from build123d import *

# Parameters (mm, degrees)
SKETCH1_R           = 9.5
BOSS_EXTRUDE1_DEPTH = 2.25


with BuildPart() as part:
    # Sketch1 → Boss-Extrude1 (new body)
    with BuildSketch(Plane(origin=(0, 0, 0), x_dir=(1, 0, 0), z_dir=(0, 1, 0))):
        Circle(SKETCH1_R)
        with BuildLine():
            ThreePointArc((-2.050056302, -4.013405112), (-0.801449739, -2.21696931), (0.006631996, -4.249997556))
            ThreePointArc((0.006631996, -4.249997556), (-1.028537661, -4.191035191), (-2.050056302, -4.013405112))
        make_face(mode=Mode.SUBTRACT)
        with BuildLine():
            ThreePointArc((7.644442426, 0), (5.613326884, -2.284952828), (2.934499964, -3.758155497))
            ThreePointArc((2.934499964, -3.758155497), (0, 3.643549808), (-2.934499964, -3.758155497))
            ThreePointArc((-2.934499964, -3.758155497), (-5.613326884, -2.284952828), (-7.644442426, 0))
            ThreePointArc((-7.644442426, 0), (0, 4.25), (7.644442426, 0))
        make_face(mode=Mode.SUBTRACT)
    extrude(amount=BOSS_EXTRUDE1_DEPTH)


solid = part.part
Geometry: final body of the model. Coordinates: model frame, mm. A direction names the side the tool comes from. Give positions to 0.01 mm unless a question says otherwise; leave off trailing zeros. Write each loop counter-clockwise with the first axis right and the second up, starting at its lowest first coordinate (ties: lowest second). Pieces come first, ordered by that corner, then holes. Notation, with made-up numbers: (-37, 82.25) -> (-18, 82.25) arc R24 ccw to (-18, 107.25) -> close; hole circle Ø10 at (32.25, 70.5). An arc over 180 degrees is marked (long way). Answer in a Markdown table with one row per item.
(1) Draft query along Z for faces 3 (the cylindrical face through (-5.58, 1.11, 2.31)), 4 (the flat face through (0, 0, 0)), 5 (the cylindrical face through (4.38, 1.11, 8.43)). Return one class per face: +Z half, -Z half, draft (parallel to the pull), parting line (faces both ways), or undercut.
Answers below:
| item | result |
|---|---|
| face 3 | undercut |
| face 4 | draft |
| face 5 | parting line |
(2) Section query A-A on y = 0.4. Return loops of the section in (x, z), then the cut area to 3 significant figures.
Answers below:
| item | result |
|---|---|
| outline | circle Ø19 at (0, 0); hole (-7.64, 0) arc R9 ccw to (7.64, 0) arc R9 ccw to (2.93, 3.76) arc R4.28 cw (long way) to (-2.93, 3.76) arc R9 ccw to start; hole (-2.05, 4.01) arc R1.24 ccw (long way) to (0.01, 4.25) arc R9 ccw to start |
| area | 242 mm^2 |
(3) Section query D-D on x = 8.5. Return loops of the section in (y, z).
Answers below:
| item | result |
|---|---|
| outline | (0, -4.24) -> (2.25, -4.24) -> (2.25, 4.24) -> (0, 4.24) -> close |
(4) Section query B-B on z = 3.25. Return loops of the section in (x, y).
Answers below:
| item | result |
|---|---|
| outline | (-8.93, 0) -> (-4.12, 0) -> (-4.12, 2.25) -> (-8.93, 2.25) -> close; (-3.39, 0) -> (-2.17, 0) -> (-2.17, 2.25) -> (-3.39, 2.25) -> close; (0.28, 0) -> (3.39, 0) -> (3.39, 2.25) -> (0.28, 2.25) -> close; (4.12, 0) -> (8.93, 0) -> (8.93, 2.25) -> (4.12, 2.25) -> close |
(5) Pin query (flat end, axial travel): pin 1 (1 mm diameter, centred on x = 4, y = 0.5, fed in from +Z). Return the tip coordinate at first contact, or that it passes through.
Answers below:
| item | result |
|---|---|
| pin 1 | z = 8.83 |
(6) Section query C-C on z = 1. Return loops of the section in (x, y).
Answers below:
| item | result |
|---|---|
| outline | (-9.45, 0) -> (-6.92, 0) -> (-6.92, 2.25) -> (-9.45, 2.25) -> close; (-4.27, 0) -> (4.27, 0) -> (4.27, 2.25) -> (-4.27, 2.25) -> close; (6.92, 0) -> (9.45, 0) -> (9.45, 2.25) -> (6.92, 2.25) -> close |
(7) Set-up query: faces 1 (the cylindrical face through (-1.014, 1.109, 4.193)), 2 (the flat face through (0, 2.25, 0)). Return all of +Z, -Z, +X, -X, +Y, -Y with unobstructed straight access to the full face (end or side cutting, diameter ignored); none if empty.
Answers below:
| item | result |
|---|---|
| face 1 | +Y, -Y |
| face 2 | +Z, -Z, +X, -X, +Y |
(8) Ray query, line 1 along X through (y, z) = (1.4, 3); line 2 along X through (y, z) = (1.9, -1); line 3 along X through (y, z) = (1.15, -0.75). Return the intervals inside material, ascending. Write a range as [from, to].
Answers below:
| item | result |
|---|---|
| line 1 | [-9.01, -4.58], [-3.57, -2.1], [0.21, 3.57], [4.58, 9.01] |
| line 2 | [-9.45, -6.92], [-3.96, 3.96], [6.92, 9.45] |
| line 3 | [-9.47, -7.12], [-4.05, 4.05], [7.12, 9.47] |
